```python
from build123d import *

# Parameters (mm, degrees)
ESQUISSE1_W             = 55
ESQUISSE1_H             = 47
BOSS_EXTRU_1_DEPTH      = 37
ESQUISSE2_R             = 2
ENL_V_MAT_EXTRU_1_DEPTH = 82.258845672
ESQUISSE3_W             = 50
ESQUISSE3_H             = 45
ENL_V_MAT_EXTRU_2_DEPTH = 1
ESQUISSE4_W             = 48
ESQUISSE4_H             = 43
ENL_V_MAT_EXTRU_3_DEPTH = 10
ESQUISSE5_R             = 10
ENL_V_MAT_EXTRU_4_DEPTH = 40
ESQUISSE6_W             = 20
ESQUISSE6_H             = 20
ENL_V_MAT_EXTRU_5_DEPTH = 10
ESQUISSE7_W             = 5
ESQUISSE7_H             = 20
ENL_V_MAT_EXTRU_6_DEPTH = 4
ESQUISSE10_R            = 2.5
ENL_V_MAT_EXTRU_7_DEPTH = 72.95832127
ENL_V_MAT_EXTRU_8_DEPTH = 4


with BuildPart() as part:
    # Esquisse1 → Boss.-Extru.1 (new body)
    with BuildSketch(Plane.XY):
        with Locations((27.5, 23.5)):
            Rectangle(ESQUISSE1_W, ESQUISSE1_H)
    extrude(amount=BOSS_EXTRU_1_DEPTH)

    # Esquisse2 → Enlèv. mat.-Extru.1 (cut, through all)
    with BuildSketch(Plane(origin=(0, 0, 0), x_dir=(-1, 0, 0), z_dir=(0, 0, -1))):
        with Locations((-51, 43)):
            Circle(ESQUISSE2_R)
        with Locations((-7, 43)):
            Circle(ESQUISSE2_R)
        with Locations((-7, 4)):
            Circle(ESQUISSE2_R)
        with Locations((-51, 4)):
            Circle(ESQUISSE2_R)
    extrude(amount=-ENL_V_MAT_EXTRU_1_DEPTH, mode=Mode.SUBTRACT)

    # Esquisse3 → Enlèv. mat.-Extru.2 (cut)
    with BuildSketch(Plane(origin=(0, 0, 0), x_dir=(-1, 0, 0), z_dir=(0, 0, -1))):
        with Locations((-29, 23.5)):
            Rectangle(ESQUISSE3_W, ESQUISSE3_H)
    extrude(amount=-ENL_V_MAT_EXTRU_2_DEPTH, mode=Mode.SUBTRACT)

    # Esquisse4 → Enlèv. mat.-Extru.3 (cut)
    with BuildSketch(Plane(origin=(0, 0, 1), x_dir=(-1, 0, 0), z_dir=(0, 0, -1))):
        with Locations((-29, 23.5)):
            Rectangle(ESQUISSE4_W, ESQUISSE4_H)
    extrude(amount=-ENL_V_MAT_EXTRU_3_DEPTH, mode=Mode.SUBTRACT)

    # Esquisse5 → Enlèv. mat.-Extru.4 (cut)
    with BuildSketch(Plane(origin=(55, 0, 0), x_dir=(0, 0, -1), z_dir=(1, 0, 0))):
        with Locations((-24, 23.5)):
            Circle(ESQUISSE5_R)
    extrude(amount=-ENL_V_MAT_EXTRU_4_DEPTH, mode=Mode.SUBTRACT)

    # Esquisse6 → Enlèv. mat.-Extru.5 (cut)
    with BuildSketch(Plane.ZY):
        with Locations((24, 23.5)):
            Rectangle(ESQUISSE6_W, ESQUISSE6_H)
    extrude(amount=-ENL_V_MAT_EXTRU_5_DEPTH, mode=Mode.SUBTRACT)

    # Esquisse7 → Enlèv. mat.-Extru.6 (cut)
    with BuildSketch(Plane(origin=(0, 0, 11), x_dir=(-1, 0, 0), z_dir=(0, 0, -1))):
        with Locations((-7.5, 23.5)):
            Rectangle(ESQUISSE7_W, ESQUISSE7_H)
    extrude(amount=-ENL_V_MAT_EXTRU_6_DEPTH, mode=Mode.SUBTRACT)

    # Esquisse10 → Enlèv. mat.-Extru.7 (cut, through all)
    with BuildSketch(Plane(origin=(15, 0, 0), x_dir=(0, 0, -1), z_dir=(1, 0, 0))):
        with Locations((-24, 23.5)):
            Circle(ESQUISSE10_R)
        with Locations((-19.5, 28)):
            Circle(ESQUISSE10_R)
        with Locations((-19.5, 19)):
            Circle(ESQUISSE10_R)
        with Locations((-28.5, 19)):
            Circle(ESQUISSE10_R)
        with Locations((-28.5, 28)):
            Circle(ESQUISSE10_R)
    extrude(amount=-ENL_V_MAT_EXTRU_7_DEPTH, mode=Mode.SUBTRACT)

    # Esquisse11 → Enlèv. mat.-Extru.8 (cut)
    with BuildSketch(Plane.XY.offset(37)):
        Polygon((11.041451884, 43), (9.020725942, 46.5), (4.979274058, 46.5), (2.958548116, 43), (4.979274058, 39.5), (9.020725942, 39.5), align=None)
        Polygon((46.958548116, 43), (48.979274058, 39.5), (53.020725942, 39.5), (55.041451884, 43), (53.020725942, 46.5), (48.979274058, 46.5), align=None)
        Polygon((46.958548116, 4), (48.979274058, 0.5), (53.020725942, 0.5), (55.041451884, 4), (53.020725942, 7.5), (48.979274058, 7.5), align=None)
        Polygon((11.041451884, 4), (9.020725942, 7.5), (4.979274058, 7.5), (2.958548116, 4), (4.979274058, 0.5), (9.020725942, 0.5), align=None)
    extrude(amount=-ENL_V_MAT_EXTRU_8_DEPTH, mode=Mode.SUBTRACT)


solid = part.part
```
Model file for the job. Use its own axes, mm. A direction names the side the tool comes from. Coordinates: 2 decimals unless noted, no trailing zeros. Write each loop counter-clockwise with the first axis right and the second up, starting at its lowest first coordinate (ties: lowest second). Pieces come first, ordered by that corner, then holes. Notation, with made-up numbers: (46.25, -28) - (73.25, -28) arc R14 ccw to (73.25, -14) - close; hole circle Ø6 at (51, 8.25). An arc over 180 degrees is marked (long way). Use a Markdown table: item, result. Add a question column.
Item 1: Band-saw the part on D-D, the plane z = 28.5. Write the cut outline in (x, y).
Item 2: Two-plate mould, pull along X, no slides. Class faces 1 (the face through (7, 7.5, 35)), 2 (the face through (54, 41.2, 35)), 3 (the face through (0, 23, 10)), 4 (the face through (5, 23, 34)): pulls with the +X half, pulls with the -X half, needs draft (parallel to the pull), parting line crosses it, or undercut.
Item 3: Band-saw the part on B-B, the plane y = 28. Write the cut outline in (x, z).
Item 4: Band-saw the part on C-C, the plane x = 33. Write the cut outline in (y, z), and give its area (3 significant figures).
Item 5: Band-saw the part on A-A, the plane z = 24. Write the cut outline in (x, y), and give its area (3 significant figures).
Item 6: Drill centre lines: line 1 along Y through (x, z) = (7, 19); line 2 along Z through (x, y) = (3.5, 27); line 3 along X through (y, z) = (41.5, 16.5). Where is each one in solid material? Low to high.
Item 7: 3-axis set-ups, long thin cutter, end or side, ignore diameter. For faces 5 (the face through (35.28, 26.5, 14.46)), 6 (the face through (51, 46.5, 35)), 7 (the face through (5, 23, 7)), 8 (the face through (13, 21, 21)): which of +Z, -Z, +X, -X, +Y, -Y reach the whole face in a straight line?
Item 8: Drop flat-ended pins along their axis: pin 1 (1 mm diameter, centred on x = 6.5, y = 3.5, fed in from -Z); pin 2 (3.5 mm diameter, centred on x = 7, y = 3.5, fed in from +Z); pin 3 (6.5 mm diameter, centred on y = 19, z = 28.5, fed in from +X). Give the stop position or say it passes through.
A:
| question | item | result |
|---|---|---|
| 1 | outline | (0, 0) - (55, 0) - (55, 14.57) - (15, 14.57) - (15, 16.5) - (10, 16.5) - (10, 13.5) - (0, 13.5) - close; (0, 33.5) - (10, 33.5) - (10, 30.5) - (15, 30.5) - (15, 32.43) - (55, 32.43) - (55, 47) - (0, 47) - close; (10, 21.5) - (15, 21.5) - (15, 25.5) - (10, 25.5) - close; hole circle Ø4 at (7, 4); hole circle Ø4 at (7, 43); hole circle Ø4 at (51, 4); hole circle Ø4 at (51, 43) |
| 2 | face 1 | undercut |
| 2 | face 2 | undercut |
| 2 | face 3 | pulls with the -X half |
| 2 | face 4 | needs draft |
| 3 | outline | (0, 0) - (4, 0) - (4, 1) - (5, 1) - (5, 14) - (0, 14) - close; (0, 34) - (10, 34) - (10, 31) - (15, 31) - (15, 32.93) - (55, 32.93) - (55, 37) - (0, 37) - close; (10, 11) - (53, 11) - (53, 1) - (54, 1) - (54, 0) - (55, 0) - (55, 15.07) - (15, 15.07) - (15, 17) - (10, 17) - close; (10, 22) - (15, 22) - (15, 26) - (10, 26) - close |
| 4 | outline | (0, 0) - (1, 0) - (1, 1) - (2, 1) - (2, 11) - (45, 11) - (45, 1) - (46, 1) - (46, 0) - (47, 0) - (47, 37) - (0, 37) - close; hole circle Ø20 at (23.5, 24) |
| 4 | area | 950 mm² |
| 5 | outline | (0, 0) - (55, 0) - (55, 13.5) - (15, 13.5) - (15, 21) - (10, 21) - (10, 13.5) - (0, 13.5) - close; (0, 33.5) - (10, 33.5) - (10, 26) - (15, 26) - (15, 33.5) - (55, 33.5) - (55, 47) - (0, 47) - close; hole circle Ø4 at (7, 4); hole circle Ø4 at (7, 43); hole circle Ø4 at (51, 4); hole circle Ø4 at (51, 43) |
| 5 | area | 1,510 mm² |
| 6 | line 1 | y = 0 to 2, 6 to 13.5, 33.5 to 41, 45 to 47 |
| 6 | line 2 | z = 0 to 14, 34 to 37 |
| 6 | line 3 | x = 0 to 5.68, 8.32 to 49.68, 52.32 to 55 |
| 7 | face 5 | +X |
| 7 | face 6 | +Z |
| 7 | face 7 | -Z |
| 7 | face 8 | +X, -X |
| 8 | pin 1 | passes through |
| 8 | pin 2 | stops at z = 33 |
| 8 | pin 3 | stops at x = 15 |
